Input: dimensioned drawing with shaded views. Units: mm. Origin: part minimum x, y, z. A direction names the side the tool comes from. Coordinates: 2 decimals unless noted, no trailing zeros. Write each loop counter-clockwise with the first axis right and the second up, starting at its lowest first coordinate (ties: lowest second). Pieces come first, ordered by that corner, then holes. Notation, with made-up numbers: M -32.5,-6 L 13.5,-6 A23 cw 13.5,7 Z; hole C 8.5,83 d4. An arc over 180 degrees is marked long. Use one line per item in the form item = value.
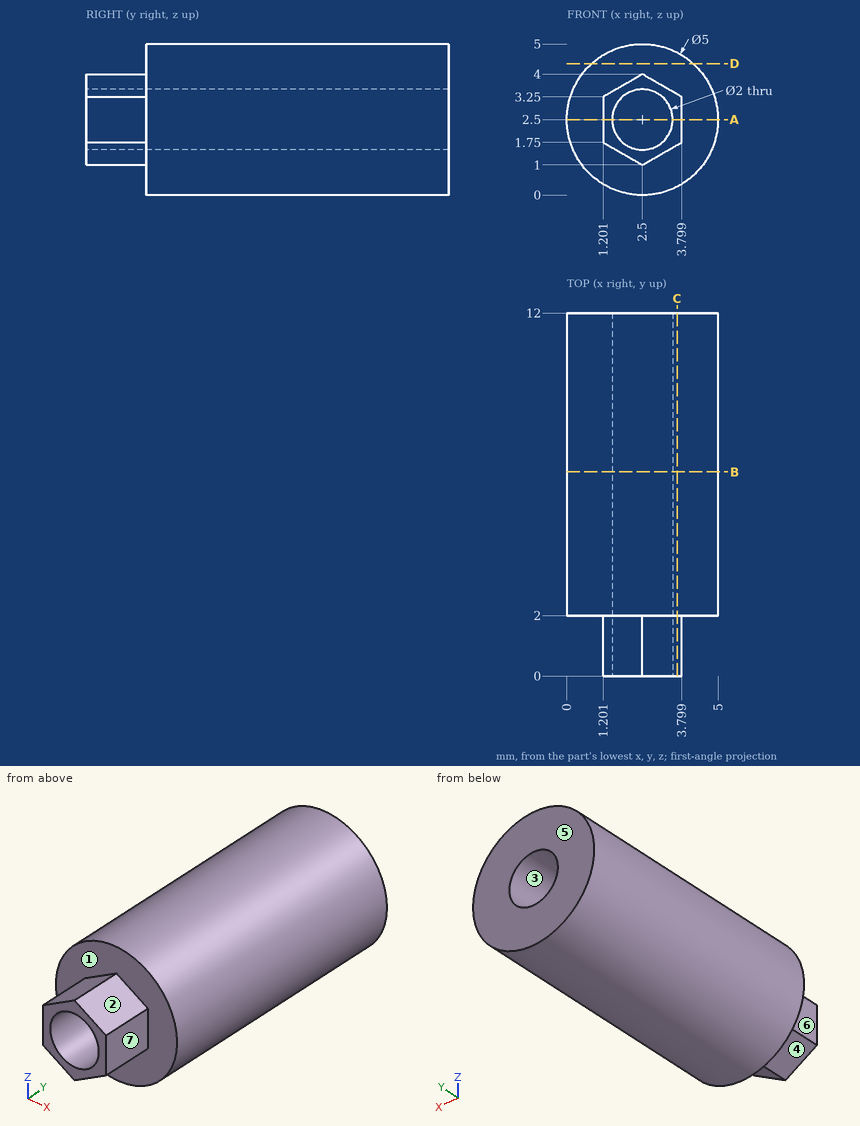
(1) Section query A-A on z = 2.5. Return the cut outline in (x, y), plus the area to 3 significant figures.
Computed:
outline = M 0,2 L 1.2,2 L 1.2,0 L 1.5,0 L 1.5,12 L 0,12 Z; M 3.5,0 L 3.8,0 L 3.8,2 L 5,2 L 5,12 L 3.5,12 Z
area = 31.2 mm^2
(2) Section query D-D on z = 4.35. Return the cut outline in (x, y).
Computed:
outline = M 0.82,2 L 4.18,2 L 4.18,12 L 0.82,12 Z
(3) Section query C-C on x = 3.65. Return the cut outline in (y, z).
Computed:
outline = M 0,1.66 L 2,1.66 L 2,0.28 L 12,0.28 L 12,4.72 L 2,4.72 L 2,3.34 L 0,3.34 Z
(4) Line query: probe 1 along X at (y, z) = (9, 2.5); probe 2 along Y at (x, z) = (0.4, 2.85). Output: solid intervals per line, ascending.
Computed:
probe_1 = 0 to 1.5, 3.5 to 5
probe_2 = 2 to 12
(5) Set-up query: the marked faces 5, 6 and 7. Return all of +Z, -Z, +X, -X, +Y, -Y with unobstructed straight access to the full face (end or side cutting, diameter ignored); none if empty.
Computed:
face_5 = +Z, -Z, +X, -X, +Y
face_6 = +Z, -Z, -X, -Y
face_7 = +Z, -Z, +X, -Y
(6) Section query B-B on y = 6.75. Return the cut outline in (x, z).
Computed:
outline = C 2.5,2.5 d5; hole C 2.5,2.5 d2
(7) Pull-direction query (Z, two-part tool) for the marked faces 1, 2, 3 and 4; classes: pulls with the +Z half, pulls with the -Z half, needs draft (parallel to the pull), parting line crosses it, or undercut.
Computed:
face_1 = needs draft
face_2 = pulls with the +Z half
face_3 = undercut
face_4 = pulls with the -Z half
(8) First-contact query: pin 1 Ø1.5 at (x, z) = (4.5, 4) entering from -Y; pin 2 Ø1.6 at (y, z) = (1.5, 2.5) entering from -X; pin 3 Ø1.8 at (x, z) = (2.5, 2.5) entering from -Y; pin 4 Ø0.8 at (y, z) = (1, 2) entering from +X. Flat tips, straight axial feed; report the tip coordinate or a pass-through.
Computed:
pin_1 = 2
pin_2 = 0
pin_3 = through
pin_4 = 3.8
